Geometry check sheet. Reference: the model listing, model coordinates, mm. A direction names the side the tool comes from. Give positions to 0.01 mm unless a question says otherwise; leave off trailing zeros. Write each loop counter-clockwise with the first axis right and the second up, starting at its lowest first coordinate (ties: lowest second). Pieces come first, ordered by that corner, then holes. Notation, with made-up numbers: (-35.75, 22) -> (2.25, 22) arc R13 cw to (2.25, 39) -> close; hole circle Ø1 at (3, 25.25). An arc over 180 degrees is marked (long way). Use a Markdown table: item, result. Add a question column.
from build123d import *

# Parameters (mm, degrees)
F0_R     = 74.1352209334
F1_DEPTH = 118.364
F3_DEPTH = 104.394
F4_R     = 16.3171471284
F5_DEPTH = 101.092
F6_R     = 17.1698744157
F7_DEPTH = 178.054


with BuildPart() as f1:
    # F0 (on Top) → F1 (new body)
    with BuildSketch(Plane.XY):
        Circle(F0_R)
    extrude(amount=F1_DEPTH)

    # F2 (on face) → F3 (join)
    with BuildSketch(Plane.XY.offset(118.364)):
        Polygon((-0.0639286038, -52.6971781414), (43.9794872102, -7.9233831007), (15.0072416542, 47.8002580793), (-46.9420066437, 37.4655672647), (-56.2565021134, -24.645264102), align=None)
    extrude(amount=F3_DEPTH)

    # F4 (on face) → F5 (join)
    with BuildSketch(Plane(origin=(26.312535727, -25.8833085534, 0), x_dir=(0.7012682501, 0.7128974971, 0), z_dir=(0.7128974971, -0.7012682501, 0))):
        with Locations((-7.3910155334, 181.9214969873)):
            Circle(F4_R)
    extrude(amount=F5_DEPTH)

    # F6 (on face) → F7 (join)
    with BuildSketch(Plane(origin=(-21.0716275073, -42.2099175124, 0), x_dir=(0.894709617, -0.4466482971, 0), z_dir=(-0.4466482971, -0.894709617, 0))):
        with Locations((0, 167.5989925861)):
            Circle(F6_R)
    extrude(amount=F7_DEPTH)


solid = f1.part
1) Draft check along Z on faces 1 (the face through (-7, -2, 222.758)), 2 (the face through (21.649, -30.624, 158.231)), 3 (the face through (29.696, 19.548, 169.83)). Enter one of: +Z half, -Z half, draft (parallel to the pull), parting line (faces both ways), or undercut.
2) Tool access check on faces 4 (the face through (93.037, -102.208, 182.15)), 5 (the face through (32, 18, 118.364)), 6 (the face through (-15.534, 42.705, 169.83)). Record the directions out of +Z, -Z, +X, -X, +Y, -Y that give a thin tool (end or side, any length) a straight path to the whole face; none if there is none.
3) Sectioned sample at C-C, the plane z = 57. Enter the section's corners in (x, y), and give its area (3 significant figures).
4) Sectioned sample at B-B, the plane y = 0. Enter the section's corners in (x, z), and give its area (3 significant figures).
5) Material ranges on probe 1 along Z at (x, y) = (-68, 9); probe 2 along X at (y, z) = (-64, 177.5); probe 3 along Y at (x, z) = (-62, 178.5), recorded low to high. Write a range as [from, to].
6) Gauge pin test, flat ends, axial feed: P1, Ø12, axis at y = 36.5, z = 157.5, coming from the +X side; P2, Ø2, axis at y = 0.5, z = 130, coming from the -X side; P3, Ø1.5, axis at x = -21.5, z = 136.5, coming from the -Y side. Record the tip position at first contact, or that the pin passes through.
7) Sectioned sample at A-A, the plane z = 206. Enter the section's corners in (x, y), and give its area (3 significant figures).
8) Sectioned sample at D-D, the plane y = 30.5. Enter the section's corners in (x, z), and give its area (3 significant figures).
Check values:
| question | item | result |
|---|---|---|
| 1 | face 1 | +Z half |
| 1 | face 2 | undercut |
| 1 | face 3 | draft |
| 2 | face 4 | +Z, -Z, +X, -Y |
| 2 | face 5 | none |
| 2 | face 6 | +Z, -X, +Y |
| 3 | outline | circle Ø148.27 at (0, 0) |
| 3 | area | 17,300 mm² |
| 4 | outline | (-74.14, 0) -> (74.14, 0) -> (74.14, 118.36) -> (39.86, 118.36) -> (39.86, 222.76) -> (-52.56, 222.76) -> (-52.56, 118.36) -> (-74.14, 118.36) -> close |
| 4 | area | 27,200 mm² |
| 5 | probe 1 | [0, 118.36] |
| 5 | probe 2 | [-47.63, -16.27], [32.12, 76.92] |
| 5 | probe 3 | [-153.9, -94.5] |
| 6 | P1 | x = 24 |
| 6 | P2 | x = -52.64 |
| 6 | P3 | y = -42.37 |
| 7 | outline | (-56.26, -24.65) -> (-0.06, -52.7) -> (43.98, -7.92) -> (15.01, 47.8) -> (-46.94, 37.47) -> close |
| 7 | area | 6,790 mm² |
| 8 | outline | (-67.57, 0) -> (67.57, 0) -> (67.57, 118.36) -> (24, 118.36) -> (24, 222.76) -> (-47.99, 222.76) -> (-47.99, 118.36) -> (-67.57, 118.36) -> close |
| 8 | area | 23,500 mm² |
